The model under review builds one solid part; all positions refer to its coordinate system, in mm. Face numbers are marked on the shaded views. A direction names the side the tool comes from. Give positions to 0.01 mm unless a question says otherwise; leave off trailing zeros. Order: outer loops, then holes, each group sorted by start corner. A loop starts at its lowest first (then second) coordinate and runs counter-clockwise, first axis right, second up.
```python
from build123d import *

# Parameters (mm, degrees)
SKETCH_W        = 220
SKETCH_H        = 40
PAD_DEPTH       = 10
SKETCH001_R     = 19
POCKET_DEPTH    = 10
PAD001_DEPTH    = 220
PAD002_DEPTH    = 220
SKETCH004_R     = 1.325
POCKET001_DEPTH = 10
SKETCH005_R     = 1.9
POCKET002_DEPTH = 10
SKETCH006_W     = 106.6
SKETCH006_H     = 10
PAD003_DEPTH    = 70
SKETCH007_W     = 19.8
SKETCH007_H     = 10
POCKET003_DEPTH = 30
SKETCH008_W     = 56.7
SKETCH008_H     = 10
PAD004_DEPTH    = 8
SKETCH009_W     = 56.7
SKETCH009_H     = 8
PAD005_DEPTH    = 20
SKETCH010_R     = 2.375
POCKET004_DEPTH = 10
POCKET005_DEPTH = 4
FILLET_R        = 5
SKETCH012_R     = 1.75
POCKET006_DEPTH = 8
SKETCH013_R     = 2.875
POCKET007_DEPTH = 4
SKETCH014_R     = 1.325
POCKET008_DEPTH = 10
SKETCH015_W     = 72
SKETCH015_H     = 7
POCKET009_DEPTH = 10
FILLET001_R     = 2
SKETCH016_W     = 220
SKETCH016_H     = 10
PAD006_DEPTH    = 3
CHAMFER_SIZE    = 2.99


with BuildPart() as part:
    # Sketch → Pad (new body)
    with BuildSketch(Plane.XY):
        Rectangle(SKETCH_W, SKETCH_H)
    extrude(amount=PAD_DEPTH)

    # Sketch001 (on Face6 of Pad) → Pocket (cut)
    with BuildSketch(Plane.XY.offset(10)):
        with Locations((-80, 0)):
            Circle(SKETCH001_R)
        with Locations((-40, 0)):
            Circle(SKETCH001_R)
        Circle(SKETCH001_R)
        with Locations((40, 0)):
            Circle(SKETCH001_R)
        with Locations((80, 0)):
            Circle(SKETCH001_R)
    extrude(amount=-POCKET_DEPTH, mode=Mode.SUBTRACT)

    # Sketch002 (on Face3 of Pocket) → Pad001 (join)
    with BuildSketch(Plane.YZ.offset(110)):
        Polygon((-10, 0), (-20, 0), (-20, 10), align=None)
    extrude(amount=-PAD001_DEPTH)

    # Sketch003 (on Face3 of Pad001) → Pad002 (join)
    with BuildSketch(Plane.YZ.offset(110)):
        Polygon((20, 10), (10, 0), (20, 0), align=None)
    extrude(amount=-PAD002_DEPTH)

    # Sketch004 (on Face5 of Pad002) → Pocket001 (cut)
    with BuildSketch(Plane.XY.offset(10)):
        with Locations((-96, 16)):
            Circle(SKETCH004_R)
        with Locations((-96, -16)):
            Circle(SKETCH004_R)
        with Locations((-64, -16)):
            Circle(SKETCH004_R)
        with Locations((-64, 16)):
            Circle(SKETCH004_R)
        with Locations((-56, 16)):
            Circle(SKETCH004_R)
        with Locations((-56, -16)):
            Circle(SKETCH004_R)
        with Locations((-24, -16)):
            Circle(SKETCH004_R)
        with Locations((-24, 16)):
            Circle(SKETCH004_R)
        with Locations((-16, 16)):
            Circle(SKETCH004_R)
        with Locations((-16, -16)):
            Circle(SKETCH004_R)
        with Locations((16, -16)):
            Circle(SKETCH004_R)
        with Locations((16, 16)):
            Circle(SKETCH004_R)
        with Locations((24, 16)):
            Circle(SKETCH004_R)
        with Locations((24, -16)):
            Circle(SKETCH004_R)
        with Locations((56, -16)):
            Circle(SKETCH004_R)
        with Locations((56, 16)):
            Circle(SKETCH004_R)
        with Locations((64, 16)):
            Circle(SKETCH004_R)
        with Locations((64, -16)):
            Circle(SKETCH004_R)
        with Locations((96, -16)):
            Circle(SKETCH004_R)
        with Locations((96, 16)):
            Circle(SKETCH004_R)
    extrude(amount=-POCKET001_DEPTH, mode=Mode.SUBTRACT)

    # Sketch005 (on Face5 of Pocket001) → Pocket002 (cut)
    with BuildSketch(Plane.XY.offset(10)):
        with Locations((-105, 10)):
            Circle(SKETCH005_R)
        with Locations((-105, -10)):
            Circle(SKETCH005_R)
        with Locations((105, 10)):
            Circle(SKETCH005_R)
        with Locations((105, -10)):
            Circle(SKETCH005_R)
    extrude(amount=-POCKET002_DEPTH, mode=Mode.SUBTRACT)

    # Sketch006 (on Face1 of Pocket002) → Pad003 (join)
    with BuildSketch(Plane(origin=(0, 20, 0), x_dir=(-1, 0, 0), z_dir=(0, 1, 0))):
        with Locations((0, 5)):
            Rectangle(SKETCH006_W, SKETCH006_H)
    extrude(amount=PAD003_DEPTH)

    # Sketch007 → Pocket003 (cut)
    with BuildSketch(Plane(origin=(0, 90, 0), x_dir=(-1, 0, 0), z_dir=(0, 1, 0))):
        with Locations((-43.4, 5)):
            Rectangle(SKETCH007_W, SKETCH007_H)
        with Locations((43.4, 5)):
            Rectangle(SKETCH007_W, SKETCH007_H)
    extrude(amount=-POCKET003_DEPTH, mode=Mode.SUBTRACT)

    # Sketch008 (on Face1 of Pocket003) → Pad004 (join)
    with BuildSketch(Plane(origin=(0, 20, 0), x_dir=(-1, 0, 0), z_dir=(0, 1, 0))):
        with Locations((-81.65, 5)):
            Rectangle(SKETCH008_W, SKETCH008_H)
        with Locations((81.65, 5)):
            Rectangle(SKETCH008_W, SKETCH008_H)
    extrude(amount=PAD004_DEPTH)

    # Sketch009 (on Face14 of Pad004) → Pad005 (join)
    with BuildSketch(Plane(origin=(0, 0, 0), x_dir=(1, 0, 0), z_dir=(0, 0, -1))):
        with Locations((-81.65, -24)):
            Rectangle(SKETCH009_W, SKETCH009_H)
        with Locations((81.65, -24)):
            Rectangle(SKETCH009_W, SKETCH009_H)
    extrude(amount=PAD005_DEPTH)

    # Sketch010 (on Face15 of Pad005) → Pocket004 (cut)
    with BuildSketch(Plane(origin=(0, 0, 0), x_dir=(1, 0, 0), z_dir=(0, 0, -1))):
        with Locations((-28, -75)):
            Circle(SKETCH010_R)
        with Locations((28, -75)):
            Circle(SKETCH010_R)
    extrude(amount=-POCKET004_DEPTH, mode=Mode.SUBTRACT)

    # Sketch011 (on Face87 of Pocket004) → Pocket005 (cut)
    with BuildSketch(Plane.XY.offset(10)):
        Polygon((-24.35, 72.892672), (-24.35, 77.107328), (-28, 79.214657), (-31.65, 77.107328), (-31.65, 72.892672), (-28, 70.785343), align=None)
        Polygon((31.65, 77.107328), (28, 79.214657), (24.35, 77.107328), (24.35, 72.892672), (28, 70.785343), (31.65, 72.892672), align=None)
    extrude(amount=-POCKET005_DEPTH, mode=Mode.SUBTRACT)

    # Fillet
    fillet_edges = [part.edges().sort_by_distance(p)[0] for p in [
        (53.3, 60, 5),
        (-53.3, 60, 5),
    ]]
    fillet(fillet_edges, radius=FILLET_R)

    # Sketch012 (on Face19 of Fillet) → Pocket006 (cut)
    with BuildSketch(Plane(origin=(0, 28, 0), x_dir=(-1, 0, 0), z_dir=(0, 1, 0))):
        with Locations((-90, -10)):
            Circle(SKETCH012_R)
        with Locations((-65, -10)):
            Circle(SKETCH012_R)
        with Locations((65, -10)):
            Circle(SKETCH012_R)
        with Locations((90, -10)):
            Circle(SKETCH012_R)
    extrude(amount=-POCKET006_DEPTH, mode=Mode.SUBTRACT)

    # Sketch013 (on Face19 of Pocket006) → Pocket007 (cut)
    with BuildSketch(Plane(origin=(0, 28, 0), x_dir=(-1, 0, 0), z_dir=(0, 1, 0))):
        with Locations((-90, -10)):
            Circle(SKETCH013_R)
        with Locations((-65, -10)):
            Circle(SKETCH013_R)
        with Locations((65, -10)):
            Circle(SKETCH013_R)
        with Locations((90, -10)):
            Circle(SKETCH013_R)
    extrude(amount=-POCKET007_DEPTH, mode=Mode.SUBTRACT)

    # Sketch014 (on Face17 of Pocket007) → Pocket008 (cut)
    with BuildSketch(Plane.XY.offset(10)):
        with Locations((-10, 85)):
            Circle(SKETCH014_R)
        with Locations((10, 85)):
            Circle(SKETCH014_R)
    extrude(amount=-POCKET008_DEPTH, mode=Mode.SUBTRACT)

    # Sketch015 (on Face19 of Pocket008) → Pocket009 (cut)
    with BuildSketch(Plane.XY.offset(10)):
        with Locations((0, 35.5)):
            Rectangle(SKETCH015_W, SKETCH015_H)
    extrude(amount=-POCKET009_DEPTH, mode=Mode.SUBTRACT)

    # Fillet001
    fillet001_edges = [part.edges().sort_by_distance(p)[0] for p in [
        (36, 39, 5),
        (-36, 39, 5),
        (-36, 32, 5),
        (36, 32, 5),
    ]]
    fillet(fillet001_edges, radius=FILLET001_R)

    # Sketch016 (on Face104 of Fillet001) → Pad006 (join)
    with BuildSketch(Plane.XZ.offset(20)):
        with Locations((0, 5)):
            Rectangle(SKETCH016_W, SKETCH016_H)
    extrude(amount=PAD006_DEPTH)

    # Chamfer
    chamfer_edges = [part.edges().sort_by_distance(p)[0] for p in [
        (0, -23, 0),
    ]]
    chamfer(chamfer_edges, length=CHAMFER_SIZE)


solid = part.part
```
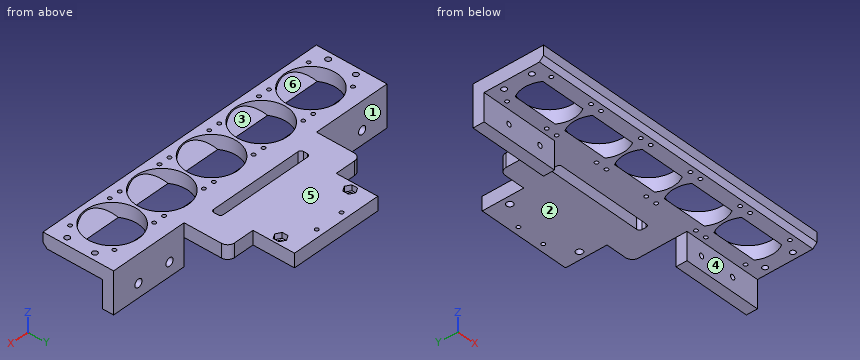
Item 1: For the marked faces 1, 2, 3 and 4, list the 3-axis set-ups (+Z, -Z, +X, -X, +Y, -Y) from which the entire face can be reached by the end or side of a thin tool; tool diameter is ignored.
Values found:
face 1: +Z, -Z, -X, +Y
face 2: -Z, -Y
face 3: +Z
face 4: -Z, +X, -X, -Y
Item 2: Take a section at D-D (x = -74). Give the boundary of the cut face in (y, z), and give its area (3 significant figures).
Values found:
outline: (-23, 2.99) - (-20.01, 0) - (-10, 0) - (-18.03, 8.03) - (-18.03, 10) - (-23, 10) - close; (10, 0) - (20, 0) - (20, -20) - (28, -20) - (28, 10) - (18.03, 10) - (18.03, 8.03) - close
area: 369 mm2
Item 3: Draft analysis for pull direction X (two halves, no side actions). For the marked faces 5 and 6, state which applies: released by +X, released by -X, zero draft, split by the parting line, or undercut.
Values found:
face 5: zero draft
face 6: undercut
Item 4: Take a section at C-C (x = -40). Give the boundary of the cut face in (y, z).
Values found:
outline: (-23, 2.99) - (-20.01, 0) - (-10, 0) - (-19, 9) - (-19, 10) - (-23, 10) - close; (10, 0) - (60, 0) - (60, 10) - (19, 10) - (19, 9) - close
Item 5: Clearance check with flat-ended pins moving along their axes: pin 1 Ø8 at (x, y) = (-11, 47.5) entering from -Z; pin 2 Ø3 at (x, y) = (56, -16) entering from +Z; pin 3 Ø6 at (x, z) = (66, -2) entering from -Y; pin 4 Ø2 at (x, z) = (-52.5, -1.5) entering from -Y. State where each tip first meets the part, or that it passes through.
Values found:
pin 1: stops at z = 0
pin 2: stops at z = 10
pin 3: stops at y = -21.01
pin 4: stops at y = 20
Item 6: Take a section at B-B (y = -2). Give the boundary of the cut face in (x, z).
Values found:
outline: (-110, 0) - (-98.89, 0) - (-98.89, 10) - (-110, 10) - close; (-61.11, 0) - (-58.89, 0) - (-58.89, 10) - (-61.11, 10) - close; (-21.11, 0) - (-18.89, 0) - (-18.89, 10) - (-21.11, 10) - close; (18.89, 0) - (21.11, 0) - (21.11, 10) - (18.89, 10) - close; (58.89, 0) - (61.11, 0) - (61.11, 10) - (58.89, 10) - close; (98.89, 0) - (110, 0) - (110, 10) - (98.89, 10) - close
Item 7: Take a section at A-A (x = 80). Give the boundary of the cut face in (y, z).
Values found:
outline: (-23, 2.99) - (-20.01, 0) - (-10, 0) - (-19, 9) - (-19, 10) - (-23, 10) - close; (10, 0) - (20, 0) - (20, -20) - (28, -20) - (28, 10) - (19, 10) - (19, 9) - close
Item 8: For line 1 (X direction, y = 85, z = 6.25) (3 decimals); line 2 (X direction, y = 12, z = 2.5); line 3 (Y direction, x = 22.5, z = 5.5), list the stretches that pass through material, from the lowest coordinate up.
Values found:
line 1: x = -33.5 to -11.325, -8.675 to 8.675, 11.325 to 33.5
line 2: x = -110 to -94.73, -65.27 to -54.73, -25.27 to -14.73, 14.73 to 25.27, 54.73 to 65.27, 94.73 to 110
line 3: y = -23 to -7.4, 7.4 to 32, 39 to 90
